For this review, take the finished solid that the model builds, in its own axes (mm). A direction names the side the tool comes from. Round coordinates to 2 decimals unless told otherwise and drop trailing zeros. Write each loop counter-clockwise with the first axis right and the second up, starting at its lowest first coordinate (ties: lowest second). Pieces come first, ordered by that corner, then holes.
from build123d import *

# Parameters (mm, degrees)
SKETCH_1_W          = 150
SKETCH_1_H          = 85
EXTRUDE_1_DEPTH     = 4
CUT_EXTRUDE_1_DEPTH = 10
SKETCH_3_R          = 1.5
CUT_EXTRUDE_2_DEPTH = 10
CUT_EXTRUDE_3_DEPTH = 10
FILLET_1_R          = 3


with BuildPart() as part:
    # 草图1 → 凸台-拉伸1 (new body)
    with BuildSketch(Plane.XY):
        Rectangle(SKETCH_1_W, SKETCH_1_H)
    extrude(amount=EXTRUDE_1_DEPTH)

    # 草图2 → 切除-拉伸1 (cut)
    with BuildSketch(Plane(origin=(0, 0, 0), x_dir=(-1, 0, 0), z_dir=(0, 0, -1))):
        Polygon((35.204977583, -42.5), (-75, 2.740355619), (-77.497943244, -0.131283493), (-84.390465543, -55.505754288), (-64.834396177, -59.115887647), align=None)
    extrude(amount=-CUT_EXTRUDE_1_DEPTH, mode=Mode.SUBTRACT)

    # 草图3 → 切除-拉伸2 (cut)
    with BuildSketch(Plane(origin=(0, 0, 0), x_dir=(-1, 0, 0), z_dir=(0, 0, -1))):
        with Locations((-60.921137183, 30.235756338)):
            Circle(SKETCH_3_R)
        with Locations((-30.921137183, 30.235756338)):
            Circle(SKETCH_3_R)
        with Locations((-0.921137183, 30.235756338)):
            Circle(SKETCH_3_R)
        with Locations((29.078862817, 30.235756338)):
            Circle(SKETCH_3_R)
        with Locations((59.078862817, 30.235756338)):
            Circle(SKETCH_3_R)
        with Locations((59.078862817, 15.004599281)):
            Circle(SKETCH_3_R)
        with Locations((29.078862817, 15.004599281)):
            Circle(SKETCH_3_R)
        with Locations((-0.921137183, 15.004599281)):
            Circle(SKETCH_3_R)
        with Locations((-30.921137183, 15.004599281)):
            Circle(SKETCH_3_R)
        with Locations((-60.921137183, 15.004599281)):
            Circle(SKETCH_3_R)
        with Locations((44.883757424, -4.600166374)):
            Circle(SKETCH_3_R)
        with Locations((44.883757424, -14.600166374)):
            Circle(SKETCH_3_R)
        with Locations((44.883757424, -24.600166374)):
            Circle(SKETCH_3_R)
        with Locations((44.883757424, -34.600166374)):
            Circle(SKETCH_3_R)
        with Locations((65.321220159, -34.600166374)):
            Circle(SKETCH_3_R)
        with Locations((65.321220159, -24.600166374)):
            Circle(SKETCH_3_R)
        with Locations((65.321220159, -14.600166374)):
            Circle(SKETCH_3_R)
        with Locations((65.321220159, -4.600166374)):
            Circle(SKETCH_3_R)
    extrude(amount=-CUT_EXTRUDE_2_DEPTH, mode=Mode.SUBTRACT)

    # 草图4 → 切除-拉伸3 (cut)
    with BuildSketch(Plane(origin=(0, 0, 0), x_dir=(-1, 0, 0), z_dir=(0, 0, -1))):
        Polygon((-34.771828022, 2.5), (35, -26.142102935), (35, 2.5), align=None)
    extrude(amount=-CUT_EXTRUDE_3_DEPTH, mode=Mode.SUBTRACT)

    # 圆角1
    fillet_1_edges = [part.edges().sort_by_distance(p)[0] for p in [
        (34.771828022, 2.5, 2),
        (-35, 2.5, 2),
        (-35, -26.142102935, 2),
        (75, 2.740355619, 2),
        (-35.204977583, -42.5, 2),
        (-75, -42.5, 2),
        (-75, 42.5, 2),
        (75, 42.5, 2),
    ]]
    fillet(fillet_1_edges, radius=FILLET_1_R)


solid = part.part
(1) Mouldability with a two-part tool opening along Y and no side actions: class faces 3 (the face through (1.246, 28.771, 1.972)), 4 (the face through (-64.13, -35.51, 1.97)), 5 (the face through (-75, -1, 2)), 6 (the face through (-1, 42.5, 2)) as pulls with the +Y half, pulls with the -Y half, needs draft (parallel to the pull), parting line crosses it, or undercut.
Geometry check:
face 3: undercut
face 4: undercut
face 5: needs draft
face 6: pulls with the +Y half
(2) We need section A-A, the plane x = -14.5. Give the boundary of the cut face in (y, z), and give its area (3 significant figures).
Geometry check:
outline: (-34, 0) - (-17.73, 0) - (-17.73, 4) - (-34, 4) - close; (2.5, 0) - (42.5, 0) - (42.5, 4) - (2.5, 4) - close
area: 225 mm2
(3) For pin 1 Ø5 at (x, y) = (-44.88, -34.6) entering from -Z; pin 2 Ø2.5 at (x, y) = (-44.88, -14.6) entering from +Z; pin 3 Ø1 at (x, z) = (12.5, 1.5) entering from -Y; pin 4 Ø1.2 at (y, z) = (-7.5, 2) entering from +X, all flat-tipped, find the tip position at first contact; note any pin that passes through.
Geometry check:
pin 1: stops at z = 0
pin 2: passes through
pin 3: stops at y = -23.12
pin 4: stops at x = 51.52
(4) We need section B-B, the plane y = -11. Give the boundary of the cut face in (x, z), and give its area (3 significant figures).
Geometry check:
outline: (-75, 0) - (-35, 0) - (-35, 4) - (-75, 4) - close; (1.89, 0) - (41.53, 0) - (41.53, 4) - (1.89, 4) - close
area: 319 mm2
(5) We need section D-D, the plane y = -31.5. Give the boundary of the cut face in (x, z).
Geometry check:
outline: (-75, 0) - (-8.41, 0) - (-8.41, 4) - (-75, 4) - close
(6) For line 1 along Y through (x, z) = (30, 3.75); line 2 along Y through (x, z) = (-24.5, 3.2); line 3 along X through (y, z) = (1, 2.45), list the stretches that pass through material, from the lowest coordinate up.
Geometry check:
line 1: y = -15.73 to 13.82, 16.19 to 29.05, 31.42 to 42.5
line 2: y = -38.11 to -21.83, 2.5 to 42.5
line 3: x = -75 to -34.6, 22.16 to 70.76
(7) For faces 1 (the face through (22.496, 0.137, 2.028)), 2 (the face through (18.486, -20.459, 1.972)), list the 3-axis set-ups (+Z, -Z, +X, -X, +Y, -Y) from which the entire face can be reached by the end or side of a thin tool; tool diameter is ignored.
Geometry check:
face 1: +Z, -Z
face 2: +Z, -Z, +X, -Y
(8) We need section C-C, the plane z = 0.9. State how many separate pieces and enclosed holes the cut face has, and give its area (3 significant figures).
Geometry check:
separate pieces: 1
enclosed holes: 19
area: 9,160 mm2
